from build123d import *

# Parameters (mm, degrees)
SKETCH1_W           = 141
SKETCH1_H           = 126
SKETCH1_W_2         = 131
SKETCH1_H_2         = 116
BOSS_EXTRUDE1_DEPTH = 10
SKETCH1_2_W         = 141
SKETCH1_2_H         = 126
SKETCH1_2_W_2       = 131
SKETCH1_2_H_2       = 116
BOSS_EXTRUDE2_DEPTH = 2


with BuildPart() as part:
    # Sketch1 → Boss-Extrude1 (new body)
    with BuildSketch(Plane(origin=(0, 0, 0), x_dir=(1, 0, 0), z_dir=(0, 1, 0))):
        with Locations((70.5, 63)):
            Rectangle(SKETCH1_W, SKETCH1_H)
        with Locations((70.5, 63)):
            Rectangle(SKETCH1_W_2, SKETCH1_H_2, mode=Mode.SUBTRACT)
    extrude(amount=-BOSS_EXTRUDE1_DEPTH)

    # Sketch1_2 → Boss-Extrude2 (add)
    # profile 1 of 2: a face of its own
    with BuildSketch(Plane(origin=(0, 0, 0), x_dir=(1, 0, 0), z_dir=(0, 1, 0))):
        with Locations((70.5, 63)):
            Rectangle(SKETCH1_2_W, SKETCH1_2_H)
        with Locations((70.5, 63)):
            Rectangle(SKETCH1_2_W_2, SKETCH1_2_H_2, mode=Mode.SUBTRACT)
    # profile 2 of 2: a face of its own
    with BuildSketch(Plane(origin=(0, 0, 0), x_dir=(1, 0, 0), z_dir=(0, 1, 0))):
        with Locations((70.5, 63)):
            Rectangle(SKETCH1_2_W_2, SKETCH1_2_H_2)
    extrude(amount=BOSS_EXTRUDE2_DEPTH)


solid = part.part
Can you work these out from the model? Positions are in its coordinate system, mm. A direction names the side the tool comes from. Round coordinates to 2 decimals unless told otherwise and drop trailing zeros. Loops run counter-clockwise (first coordinate to the right, second up) from the corner with the lowest first, then second, coordinate; pieces in that order, holes last. Notation, with made-up numbers: (83.25, 61) - (117.25, 61) arc R35 cw to (117.25, 96) - close; hole circle Ø2 at (23, 76). An arc over 180 degrees is marked (long way). Write item = value, one per line. Start each with the question number.
(1) If we section it at B-B (y = -3): Please give me the cut outline in (x, z), and give its area (3 significant figures).
(2) If we mould it in two halves opening along X, with no side actions, what happens to faces 1 (the face through (136, -5, -62)), 2 (the face through (70, 2, -64)), 3 (the face through (0, -4, -62))? For each: released by +X, released by -X, zero draft, split by the parting line, or undercut.
(3) For P1, Ø12, axis at x = 115, z = -22.5, coming from the -Y side, with a flat end and sliding along its axis, tell me the tip position at first contact or that it passes through.
(4) For faces 4 (the face through (141, -4, -62)), 5 (the face through (5, -5, -62)), which set-ups out of +Z, -Z, +X, -X, +Y, -Y let a thin tool reach every point of the face, with its end or its side?
(5) If we section it at A-A (x = 28.5): Please give me the cut outline in (y, z), and give its area (3 significant figures).
(6) If I drill on probe 1 along Z at (x, y) = (44, -9); probe 2 along X at (y, z) = (-7, -51); probe 3 along Y at (x, z) = (126.5, -22), over which ranges is the centre line in solid material (lowest first)? Write a range as [from, to].
(7) If we section it at C-C (z = -97): Please give me the cut outline in (x, y).
Ans:
q1.outline = (0, -126) - (141, -126) - (141, 0) - (0, 0) - close; hole (5, -121) - (136, -121) - (136, -5) - (5, -5) - close
q1.area = 2,570 mm²
q2.face_1 = undercut
q2.face_2 = zero draft
q2.face_3 = released by -X
q3.P1 = 0
q4.face_4 = +Z, -Z, +X, +Y, -Y
q4.face_5 = -Y
q5.outline = (-10, -126) - (2, -126) - (2, 0) - (-10, 0) - (-10, -5) - (0, -5) - (0, -121) - (-10, -121) - close
q5.area = 352 mm²
q6.probe_1 = [-126, -121], [-5, 0]
q6.probe_2 = [0, 5], [136, 141]
q6.probe_3 = [0, 2]
q7.outline = (0, -10) - (5, -10) - (5, 0) - (136, 0) - (136, -10) - (141, -10) - (141, 2) - (0, 2) - close
